CAD build for the part. Positions are in the model's coordinates, mm. A direction names the side the tool comes from. Round coordinates to 2 decimals unless told otherwise and drop trailing zeros. Order: outer loops, then holes, each group sorted by start corner. A loop starts at its lowest first (then second) coordinate and runs counter-clockwise, first axis right, second up. Notation, with made-up numbers: (30, -17.5) -> (78, -17.5) arc R32 cw to (78, 17.5) -> close; hole circle Ø7 at (-24.75, 2.5). An arc over 180 degrees is marked (long way). Return JSON: item names as keys, results as strings. Group by question number.
Q1. Flat gauge pins, fed straight in: pin 1 (3 mm diameter, centred on x = -10, y = 1, fed in from +Z); pin 2 (5 mm diameter, centred on x = -9, y = 16, fed in from -Z); pin 3 (10 mm diameter, centred on y = 4.5, z = 15.5, fed in from +X); pin 4 (14.5 mm diameter, centred on y = -12.573, z = 14.224, fed in from -X). Where does each tip first touch, or does it go through?
Q2. Cut at A-A (y = 9). Write the cut outline in (x, z), then the cut area to 3 significant figures.
Q3. Cut at B-B (z = 15.75). Write the cut outline in (x, y) (3 decimals), then the cut area to 3 significant figures.
Q4. Mould opens along Z. For faces 4 (the flat face through (-10, -15, 24.409)), 5 (the flat face through (-11.872, 0, 25)), 6 (the flat face through (-12.5, 0.4, 26.924)) say: +Z half, -Z half, draft (parallel to the pull), parting line (faces both ways), or undercut.
Q5. Probe line 1 along Z through (x, y) = (-9, 14); line 2 along Y through (x, z) = (-12.5, 9.25) (3 decimals); line 3 along Z through (x, y) = (-15.75, 1) (3 decimals). List the from-to ranges inside material, lowest first.
Q6. Cut at C-C (x = -6.25). Write the cut outline in (y, z) (3 decimals), then the cut area to 3 significant figures.
Q7. Cut at D-D (y = -14). Write the cut outline in (x, z), then the cut area to 3 significant figures.
Q8. Which spindle directions (+Z, -Z, +X, -X, +Y, -Y) get a long thin tool onto all of the face, cutting with end or side? Do faces 1 (the cylindrical face through (-17.804, -0.291, -0.73)), 2 (the flat face through (-13, 0, 4.293)), 3 (the flat face through (-8.274, 2.827, -0.682)). Say none if no direction does.
from build123d import *

# Parameters (mm, degrees)
BOSS_EXTRUDE1_DEPTH      = 1.524
BOSS_EXTRUDE1_DEPTH_BACK = 3.048
BOSS_EXTRUDE2_DEPTH      = 1.016
BOSS_EXTRUDE3_DEPTH      = 1.143
SKETCH4_W                = 6.35
SKETCH4_H                = 52.07
BOSS_EXTRUDE4_DEPTH      = 25.4
SKETCH5_W                = 20.3708
SKETCH5_H                = 46.99
CUT_EXTRUDE1_DEPTH       = 2.54
SKETCH6_R                = 8.128
CUT_EXTRUDE2_DEPTH       = 7.695152554
SKETCH7_W                = 3.302
SKETCH7_H                = 13.716
CUT_EXTRUDE3_DEPTH       = 3.048
CUT_EXTRUDE4_DEPTH       = 3.81


with BuildPart() as part:
    # Sketch1 → Boss-Extrude1 (new body, two sides)
    with BuildSketch(Plane.XY) as boss_extrude1_sk:
        with BuildLine():
            Line((-2.221121967, 3.920099398), (-14.159121967, 3.267778706))
            ThreePointArc((-14.159121967, 3.267778706), (-17.805238677, -0.371570093), (-14.172670351, -4.024442128))
            Line((-14.172670351, -4.024442128), (-2.234670351, -3.953900602))
            Line((-2.234670351, -3.953900602), (-2.209072203, -3.191900602))
            Line((-2.209072203, -3.191900602), (-14.147072203, -3.262442128))
            ThreePointArc((-14.147072203, -3.262442128), (-17.043238677, -0.384369192), (-14.159121967, 2.505778706))
            Line((-14.159121967, 2.505778706), (-2.221121967, 3.158099398))
            Line((-2.221121967, 3.158099398), (-2.221121967, 3.920099398))
        make_face()
    extrude(amount=BOSS_EXTRUDE1_DEPTH)
    extrude(boss_extrude1_sk.sketch, amount=-BOSS_EXTRUDE1_DEPTH_BACK)

    # Sketch2 → Boss-Extrude2 (add)
    with BuildSketch(Plane.XY.offset(1.524)):
        with BuildLine():
            Line((-2.209072203, -3.191900602), (-2.221121967, 3.158099398))
            Line((-2.221121967, 3.158099398), (-14.159121967, 2.505778706))
            ThreePointArc((-14.159121967, 2.505778706), (-17.043238677, -0.384369192), (-14.147072203, -3.262442128))
            Line((-14.147072203, -3.262442128), (-2.209072203, -3.191900602))
        make_face()
    extrude(amount=-BOSS_EXTRUDE2_DEPTH)

    # Sketch3 → Boss-Extrude3 (add)
    with BuildSketch(Plane(origin=(0, 0, -3.048), x_dir=(-1, 0, 0), z_dir=(0, 0, -1))):
        with BuildLine():
            Line((14.159121967, 2.505778706), (2.221121967, 3.158099398))
            Line((2.221121967, 3.158099398), (2.209072203, -3.191900602))
            Line((2.209072203, -3.191900602), (14.147072203, -3.262442128))
            ThreePointArc((14.147072203, -3.262442128), (17.043238677, -0.384369192), (14.159121967, 2.505778706))
        make_face()
    extrude(amount=-BOSS_EXTRUDE3_DEPTH)

    # Sketch4 → Boss-Extrude4 (add)
    with BuildSketch(Plane.XY.offset(1.524)):
        with Locations((-11.745092416, 0)):
            Rectangle(SKETCH4_W, SKETCH4_H)
    extrude(amount=BOSS_EXTRUDE4_DEPTH)

    # Sketch5 → Cut-Extrude1 (cut)
    with BuildSketch(Plane(origin=(-8.570092416, 0, 0), x_dir=(0, 0, -1), z_dir=(1, 0, 0))):
        with Locations((-14.224, 0)):
            Rectangle(SKETCH5_W, SKETCH5_H)
    extrude(amount=-CUT_EXTRUDE1_DEPTH, mode=Mode.SUBTRACT)

    # Sketch6 → Cut-Extrude2 (cut, through all)
    with BuildSketch(Plane(origin=(-11.110092416, 0, 0), x_dir=(0, 0, -1), z_dir=(1, 0, 0))):
        with Locations((-14.224, -12.573)):
            Circle(SKETCH6_R)
        with Locations((-14.224, 12.573)):
            Circle(SKETCH6_R)
    extrude(amount=-CUT_EXTRUDE2_DEPTH, mode=Mode.SUBTRACT)

    # Sketch7 → Cut-Extrude3 (cut)
    with BuildSketch(Plane.XY.offset(26.924)):
        with Locations((-10.221092416, 0)):
            Rectangle(SKETCH7_W, SKETCH7_H)
    extrude(amount=-CUT_EXTRUDE3_DEPTH, mode=Mode.SUBTRACT)

    # Sketch8 → Cut-Extrude4 (cut)
    with BuildSketch(Plane(origin=(-11.110092416, 0, 0), x_dir=(0, 0, -1), z_dir=(1, 0, 0))):
        with BuildLine():
            Line((-8.3566, -5.588), (-8.3566, 5.588))
            ThreePointArc((-8.3566, 5.588), (-6.3246, 7.62), (-4.2926, 5.588))
            Line((-4.2926, 5.588), (-4.2926, -5.588))
            ThreePointArc((-4.2926, -5.588), (-6.3246, -7.62), (-8.3566, -5.588))
        make_face()
    extrude(amount=-CUT_EXTRUDE4_DEPTH, mode=Mode.SUBTRACT)


solid = part.part
Solution:
{
 "1": {"pin 1": "stops at z = 23.88", "pin 2": "stops at z = 1.52", "pin 3": "stops at x = -11.11", "pin 4": "passes through"},
 "2": {"outline": "(-14.92, 1.52) -> (-8.57, 1.52) -> (-8.57, 4.04) -> (-11.11, 4.04) -> (-11.11, 6.92) -> (-14.92, 6.92) -> close; (-14.92, 21.52) -> (-11.11, 21.52) -> (-11.11, 24.41) -> (-8.57, 24.41) -> (-8.57, 26.92) -> (-14.92, 26.92) -> close", "area": "53.9 mm²"},
 "3": {"outline": "(-14.92, -26.035) -> (-8.57, -26.035) -> (-8.57, -23.495) -> (-11.11, -23.495) -> (-11.11, -20.556) -> (-14.92, -20.556) -> close; (-14.92, -4.59) -> (-11.11, -4.59) -> (-11.11, 4.59) -> (-14.92, 4.59) -> close; (-14.92, 20.556) -> (-11.11, 20.556) -> (-11.11, 23.495) -> (-8.57, 23.495) -> (-8.57, 26.035) -> (-14.92, 26.035) -> close", "area": "89.6 mm²"},
 "4": {"face 4": "undercut", "face 5": "draft", "face 6": "+Z half"},
 "5": {"line 1": "z = 1.52 to 4.04, 24.41 to 26.92", "line 2": "y = -26.035 to -19.001, -6.145 to 6.145, 19.001 to 26.035", "line 3": "z = -3.048 to -1.905, 0.508 to 1.524"},
 "6": {"outline": "(-3.978, -3.048) -> (3.7, -3.048) -> (3.7, 1.524) -> (-3.978, 1.524) -> close; hole (-3.216, -1.905) -> (2.938, -1.905) -> (2.938, 0.508) -> (-3.216, 0.508) -> close", "area": "20.3 mm²"},
 "7": {"outline": "(-14.92, 1.52) -> (-8.57, 1.52) -> (-8.57, 4.04) -> (-11.11, 4.04) -> (-11.11, 6.22) -> (-14.92, 6.22) -> close; (-14.92, 22.23) -> (-11.11, 22.23) -> (-11.11, 24.41) -> (-8.57, 24.41) -> (-8.57, 26.92) -> (-14.92, 26.92) -> close", "area": "48.6 mm²"},
 "8": {"face 1": "-Z, -X", "face 2": "+X, -X", "face 3": "+X"}
}
